Can you work these out from the model? Positions are in its coordinate system, mm. Face numbers are marked on the shaded views. A direction names the side the tool comes from. Round coordinates to 2 decimals unless told otherwise and drop trailing zeros. Loops run counter-clockwise (first coordinate to the right, second up) from the corner with the lowest first, then second, coordinate; pieces in that order, holes last.
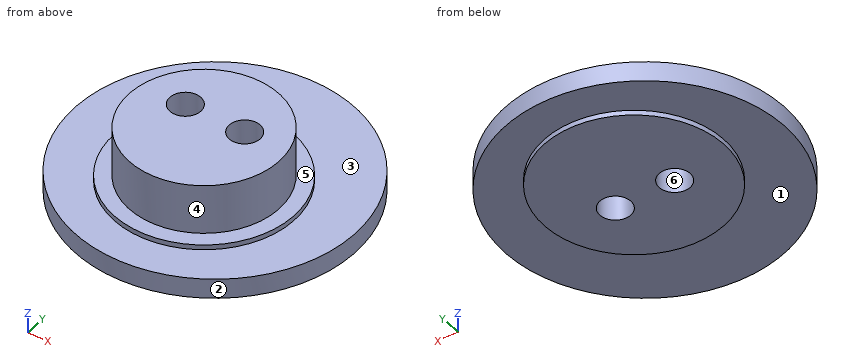
from build123d import *

# Parameters (mm, degrees)
SKETCH1_R           = 14
BOSS_EXTRUDE1_DEPTH = 2
SKETCH2_R           = 9
BOSS_EXTRUDE2_DEPTH = 0.5
SKETCH4_R           = 7.5
BOSS_EXTRUDE3_DEPTH = 5
SKETCH6_R           = 9
BOSS_EXTRUDE4_DEPTH = 0.5
SKETCH5_R           = 1.55
CUT_EXTRUDE1_DEPTH  = 22.354156504


with BuildPart() as part:
    # Sketch1 → Boss-Extrude1 (new body)
    with BuildSketch(Plane.XY):
        Circle(SKETCH1_R)
    extrude(amount=BOSS_EXTRUDE1_DEPTH)

    # Sketch2 → Boss-Extrude2 (add)
    with BuildSketch(Plane.XY.offset(2)):
        with Locations((0, -1.5)):
            Circle(SKETCH2_R)
    extrude(amount=BOSS_EXTRUDE2_DEPTH)

    # Sketch4 → Boss-Extrude3 (add)
    with BuildSketch(Plane.XY.offset(2.5)):
        with Locations((0, -1.5)):
            Circle(SKETCH4_R)
    extrude(amount=BOSS_EXTRUDE3_DEPTH)

    # Sketch6 → Boss-Extrude4 (add)
    with BuildSketch(Plane(origin=(0, 0, 0), x_dir=(-1, 0, 0), z_dir=(0, 0, -1))):
        with Locations((0, 1.5)):
            Circle(SKETCH6_R)
    extrude(amount=BOSS_EXTRUDE4_DEPTH)

    # Sketch5 → Cut-Extrude1 (cut, through all)
    with BuildSketch(Plane.XY.offset(7.5)):
        with Locations((3, 0)):
            Circle(SKETCH5_R)
        with Locations(Location((-3, 0, 0), (0, 0, 180))):
            Circle(SKETCH5_R)
    extrude(amount=-CUT_EXTRUDE1_DEPTH, mode=Mode.SUBTRACT)


solid = part.part
(1) If we mould it in two halves opening along X, with no side actions, what happens to the marked faces 4, 5 and 6? For each: released by +X, released by -X, zero draft, split by the parting line, or undercut.
Worked answers:
face 4: split by the parting line
face 5: zero draft
face 6: undercut
(2) If we section it at D-D, the plane y = -4.5: List the corners of the cut face in (x, z) for me.
Worked answers:
outline: (-13.26, 0) - (-6.71, 0) - (-6.71, -0.5) - (6.71, -0.5) - (6.71, 0) - (13.26, 0) - (13.26, 2) - (8.49, 2) - (8.49, 2.5) - (6.87, 2.5) - (6.87, 7.5) - (-6.87, 7.5) - (-6.87, 2.5) - (-8.49, 2.5) - (-8.49, 2) - (-13.26, 2) - close
(3) If we section it at A-A, the plane x = -2.75: List the corners of the cut face in (y, z) for me, then the cut area to 3 significant figures.
Worked answers:
outline: (-13.73, 0) - (-7.07, 0) - (-7.07, -0.5) - (-1.53, -0.5) - (-1.53, 7.5) - (-8.48, 7.5) - (-8.48, 2.5) - (-10.07, 2.5) - (-10.07, 2) - (-13.73, 2) - close; (1.53, -0.5) - (10.07, -0.5) - (10.07, 0) - (13.73, 0) - (13.73, 2) - (7.07, 2) - (7.07, 2.5) - (5.48, 2.5) - (5.48, 7.5) - (1.53, 7.5) - close
area: 117 mm2
(4) If we section it at C-C, the plane x = -7: List the corners of the cut face in (y, z) for me.
Worked answers:
outline: (-12.12, 0) - (-4.16, 0) - (-4.16, -0.5) - (7.16, -0.5) - (7.16, 0) - (12.12, 0) - (12.12, 2) - (4.16, 2) - (4.16, 2.5) - (1.19, 2.5) - (1.19, 7.5) - (-4.19, 7.5) - (-4.19, 2.5) - (-7.16, 2.5) - (-7.16, 2) - (-12.12, 2) - close
(5) If I drill on line 1 (Z direction, x = -9, y = -5.25); line 2 (Z direction, x = -4.25, y = 7.75); line 3 (Y direction, x = -3, z = 4.5), over which ranges is the centre line in solid material (lowest first)?
Worked answers:
line 1: z = 0 to 2
line 2: z = -0.5 to 2
line 3: y = -8.37 to -1.55, 1.55 to 5.37
(6) For the marked faces 1, 2 and 3, which set-ups out of +Z, -Z, +X, -X, +Y, -Y let a thin tool reach every point of the face, with its end or its side?
Worked answers:
face 1: -Z
face 2: +Z, -Z
face 3: +Z
(7) Will these pins go through, and if not, where does the flat tip stop? P1, Ø2, axis at x = -2, z = 2.5, coming from the +Y side; P2, Ø8, axis at x = 9.5, y = -10.5, coming from the -Z side; P3, Ø1, axis at y = -3.5, z = 5, coming from the -X side.
Worked answers:
P1: stops at y = 13.95
P2: stops at z = 0
P3: stops at x = -7.35
(8) If we section it at B-B, the plane y = 1: List the corners of the cut face in (x, z) for me.
Worked answers:
outline: (-13.96, 0) - (-8.99, 0) - (-8.99, -0.5) - (-4.18, -0.5) - (-4.18, 7.5) - (-7.07, 7.5) - (-7.07, 2.5) - (-8.65, 2.5) - (-8.65, 2) - (-13.96, 2) - close; (-1.82, -0.5) - (1.82, -0.5) - (1.82, 7.5) - (-1.82, 7.5) - close; (4.18, -0.5) - (8.99, -0.5) - (8.99, 0) - (13.96, 0) - (13.96, 2) - (8.65, 2) - (8.65, 2.5) - (7.07, 2.5) - (7.07, 7.5) - (4.18, 7.5) - close
